Verification items for the finished model (mm, model axes). Give positions to 0.01 mm unless a question says otherwise; leave off trailing zeros. Write each loop counter-clockwise with the first axis right and the second up, starting at its lowest first coordinate (ties: lowest second). Pieces come first, ordered by that corner, then holes. Notation, with made-up numbers: (13.5, -26) -> (50.5, -26) arc R22 cw to (50.5, -20) -> close; hole circle Ø10 at (-18.5, -12.75). An arc over 180 degrees is marked (long way). Use one line per item in the form item = value. Start each with the question number.
(1) Section check C-C, the plane z = 5.5. Record the cut outline in (x, y), plus the area to 3 significant figures.
(2) Scan lines: L1, parallel to X at y = 1, z = 10; L2, parallel to X at y = 17, z = 5.5; L3, parallel to X at y = 20, z = 10.75. Record each from-to range of solid material in increasing order.
(3) Section check A-A, the plane y = 0. Record the cut outline in (x, z), plus the area to 3 significant figures.
(4) Depth check by flat-ended pin: pin 1 Ø6 at (x, y) = (1, 39) entering from +Z; pin 2 Ø4 at (y, z) = (3, 6.5) entering from -X; pin 3 Ø1 at (y, z) = (38.5, 7) entering from -X. Enter the tip coordinate at first touch or a pass-through.
(5) Release check for a two-part mould opening along X. For faces 1 (the face through (38, -21, 17)), 2 (the face through (47.69, 15.02, 8.42)), 3 (the face through (-8.67, -39.05, 8.42)), 4 (the face through (-40.768, 20.775, 8.381)) record: pulls with the +X half, pulls with the -X half, needs draft (parallel to the pull), parting line crosses it, or undercut.
from build123d import *

# Parameters (mm, degrees)
F0_R     = 50
F0_R_2   = 2.2916267838
F0_R_3   = 40
F1_DEPTH = 17


# Not quite as in the source:
# - a fillet or chamfer that OpenCascade refuses, or shapes differently, is made with other operations: its cross-section is extruded or revolved along the edge and cut away or added


with BuildPart() as f1:
    # F0 (on Top) → F1 (new body)
    with BuildSketch(Plane.XY):
        Circle(F0_R)
        with Locations((-40.46940431, 18.5024235398)):
            Circle(F0_R_2, mode=Mode.SUBTRACT)
        Circle(F0_R_3, mode=Mode.SUBTRACT)
    extrude(amount=F1_DEPTH)

    # F2: fillet of radius 3 on 5 edges, made by hand

    # F2_s1 → F2_t2 (revolve, cut)
    with BuildSketch(Plane.XZ):
        with BuildLine():
            ThreePointArc((50, 3), (49.1213203436, 0.8786796564), (47, 0))
            Line((47, 0), (50, 0))
            Line((50, 0), (50, 3))
        make_face()
    revolve(axis=Axis((0, 0, 0), (0, 0, 1)), mode=Mode.SUBTRACT)

    # F2_s3 → F2_t4 (revolve, cut)
    with BuildSketch(Plane.XZ):
        with BuildLine():
            ThreePointArc((50, 14), (49.1213203436, 16.1213203436), (47, 17))
            Line((47, 17), (50, 17))
            Line((50, 17), (50, 14))
        make_face()
    revolve(axis=Axis((0, 0, 17), (0, 0, 1)), mode=Mode.SUBTRACT)

    # F2_s5 → F2_t6 (revolve, cut)
    with BuildSketch(Plane.XZ):
        with BuildLine():
            ThreePointArc((40, 14), (40.8786796564, 16.1213203436), (43, 17))
            Line((43, 17), (40, 17))
            Line((40, 17), (40, 14))
        make_face()
    revolve(axis=Axis((0, 0, 17), (0, 0, 1)), mode=Mode.SUBTRACT)

    # F2_s7 → F2_t8 (revolve, cut)
    with BuildSketch(Plane.XZ):
        with BuildLine():
            ThreePointArc((40, 3), (40.8786796564, 0.8786796564), (43, 0))
            Line((43, 0), (40, 0))
            Line((40, 0), (40, 3))
        make_face()
    revolve(axis=Axis((0, 0, 0), (0, 0, 1)), mode=Mode.SUBTRACT)


solid = f1.part
Completed:
q1.outline = circle Ø100 at (0, 0); hole circle Ø4.58 at (-40.47, 18.5); hole circle Ø80 at (0, 0)
q1.area = 2,810 mm²
q2.L1 = -49.99 to -39.99, 39.99 to 49.99
q2.L2 = -47.02 to -42.2, -38.74 to -36.21, 36.21 to 47.02
q2.L3 = -45.83 to -42.2, -38.73 to -34.64, 34.64 to 45.83
q3.outline = (-50, 3) arc R3 ccw to (-47, 0) -> (-43, 0) arc R3 ccw to (-40, 3) -> (-40, 14) arc R3 ccw to (-43, 17) -> (-47, 17) arc R3 ccw to (-50, 14) -> close; (40, 3) arc R3 ccw to (43, 0) -> (47, 0) arc R3 ccw to (50, 3) -> (50, 14) arc R3 ccw to (47, 17) -> (43, 17) arc R3 ccw to (40, 14) -> close
q3.area = 325 mm²
q4.pin_1 = 16.83
q4.pin_2 = -49.99
q4.pin_3 = -32.5
q5.face_1 = needs draft
q5.face_2 = parting line crosses it
q5.face_3 = undercut
q5.face_4 = undercut
